The model under review builds one solid part; all positions refer to its coordinate system, in mm. Face numbers are marked on the shaded views. A direction names the side the tool comes from. Give positions to 0.01 mm unless a question says otherwise; leave off trailing zeros. Loops run counter-clockwise (first coordinate to the right, second up) from the corner with the lowest first, then second, coordinate; pieces in that order, holes last. Notation, with made-up numbers: (3.5, 16.25) - (49.5, 16.25) arc R26 cw to (49.5, 47.25) - close; hole circle Ø2 at (17, 69). An arc over 180 degrees is marked (long way). Answer as a JSON object with one key per item and string values.
from build123d import *

# Parameters (mm, degrees)
BOSS_EXTRUDE2_DEPTH      = 10
SKETCH3_R                = 3
BOSS_EXTRUDE3_DEPTH      = 100
BOSS_EXTRUDE3_DEPTH_BACK = 110
BOSS_EXTRUDE4_DEPTH      = 3
BOSS_EXTRUDE5_DEPTH      = 3
BOSS_EXTRUDE6_DEPTH      = 3
CUT_EXTRUDE1_REACH       = 22
SKETCH9_W                = 10
SKETCH9_H                = 0.75


with BuildPart() as part:
    # Sketch1 → Boss-Extrude2 (new body)
    with BuildSketch(Plane.XY):
        with BuildLine():
            Line((5, 100), (5, 0))
            Line((5, 0), (5, -10))
            Line((5, -10), (-5, -10))
            Line((-5, -10), (-5, 0))
            Line((-5, 0), (-5, 100))
            ThreePointArc((-5, 100), (0, 105), (5, 100))
        make_face()
        with BuildLine():
            Line((-2.5, 0), (-2.5, 100))
            ThreePointArc((-2.5, 100), (0, 102.5), (2.5, 100))
            Line((2.5, 100), (2.5, 0))
            ThreePointArc((2.5, 0), (0, -2.5), (-2.5, 0))
        make_face(mode=Mode.SUBTRACT)
    extrude(amount=BOSS_EXTRUDE2_DEPTH)

    # Sketch3 → Boss-Extrude3 (add, two sides)
    with BuildSketch(Plane(origin=(5, 0, 0), x_dir=(0, 0, -1), z_dir=(1, 0, 0))) as boss_extrude3_sk:
        with Locations((-5, -6.25)):
            Circle(SKETCH3_R)
    extrude(amount=BOSS_EXTRUDE3_DEPTH)
    extrude(boss_extrude3_sk.sketch, amount=-BOSS_EXTRUDE3_DEPTH_BACK)

    # Sketch6 → Boss-Extrude4 (add)
    with BuildSketch(Plane(origin=(0, -9.25, 0), x_dir=(-1, 0, 0), z_dir=(0, -1, 0))):
        Polygon((-105, -2), (-105, 10), (-135, 10), (-135, -20), (-105, -20), (-105, -8), align=None)
        Polygon((105, -2), (105, 10), (135, 10), (135, -20), (105, -20), (105, -8), align=None)
    extrude(amount=-BOSS_EXTRUDE4_DEPTH)

    # Sketch7 → Boss-Extrude5 (add)
    with BuildSketch(Plane(origin=(0, -6.25, 0), x_dir=(1, 0, 0), z_dir=(0, 1, 0))):
        Polygon((-105, -2), (-105, 10), (-135, 10), (-135, -20), (-105, -20), (-105, -8), align=None)
        Polygon((-108, -2), (-108, 7), (-132, 7), (-132, -17), (-108, -17), (-108, -8), align=None, mode=Mode.SUBTRACT)
    extrude(amount=BOSS_EXTRUDE5_DEPTH)

    # Sketch8 → Boss-Extrude6 (add)
    with BuildSketch(Plane(origin=(0, -6.25, 0), x_dir=(1, 0, 0), z_dir=(0, 1, 0))):
        Polygon((135, -2), (135, 10), (105, 10), (105, -20), (135, -20), (135, -8), align=None)
        Polygon((132, -2), (132, 7), (108, 7), (108, -17), (132, -17), (132, -8), align=None, mode=Mode.SUBTRACT)
    extrude(amount=BOSS_EXTRUDE6_DEPTH)

    # Sketch9 → Cut-Extrude1 (cut, up to next)
    with BuildSketch(Plane.XY.offset(10), mode=Mode.PRIVATE) as cut_extrude1_sk1:
        with Locations((0, -9.625)):
            Rectangle(SKETCH9_W, SKETCH9_H)
    cut_extrude1_tool1 = extrude(cut_extrude1_sk1.sketch, amount=-CUT_EXTRUDE1_REACH, mode=Mode.PRIVATE) & part.part
    add(cut_extrude1_tool1.solids().sort_by_distance((0, -9.625, 10))[0], mode=Mode.SUBTRACT)


solid = part.part
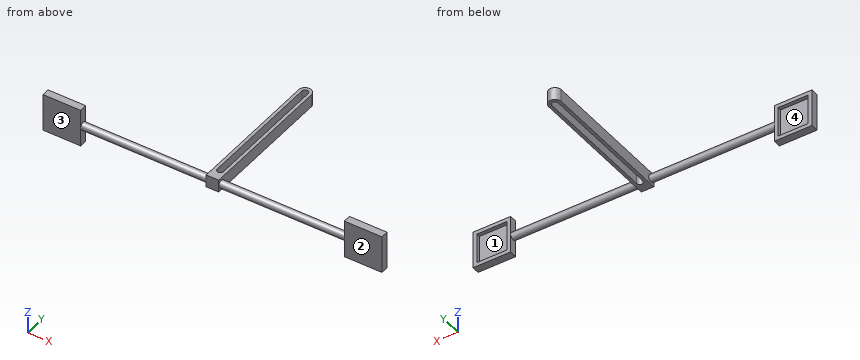
Q1. The part is to be moulded in two halves that separate along X. For the marked faces 3 and 4, say which applies: +X half, -X half, draft (parallel to the pull), parting line (faces both ways), or undercut.
Results:
{"face 3": "draft", "face 4": "undercut"}
Q2. For the marked faces 1 and 2, list the 3-axis set-ups (+Z, -Z, +X, -X, +Y, -Y) from which the entire face can be reached by the end or side of a thin tool; tool diameter is ignored.
Results:
{"face 1": "+Y", "face 2": "+Z, -Z, +X, -X, -Y"}
Q3. To check wall thickness, follow probe 1 along X at (y, z) = (31.5, 1.5); probe 2 along X at (y, z) = (-4, 17.25); probe 3 along Y at (x, z) = (116, 17.5). State the ranges of each line that lie inside material, in increasing order. Write a range as [from, to].
Results:
{"probe 1": "x = [-5, -2.5], [2.5, 5]", "probe 2": "x = [-135, -105], [105, 135]", "probe 3": "y = [-9.25, -3.25]"}
Q4. Clearance check with flat-ended pins moving along their axes: pin 1 Ø12 at (y, z) = (20, -0.5) entering from +X; pin 2 Ø12 at (x, y) = (29, 6) entering from -Z; pin 3 Ø12 at (x, z) = (123, 5.5) entering from +Y; pin 4 Ø8 at (x, z) = (-15.5, 4) entering from -Y. State where each tip first meets the part, or that it passes through.
Results:
{"pin 1": "stops at x = 5", "pin 2": "passes through", "pin 3": "stops at y = -6.25", "pin 4": "stops at y = -9.25"}
Q5. Consider section A-A, the plane x = 0. State the section outline as (y, z) points, plus the area to 3 significant figures.
Results:
{"outline": "(-9.25, 0) - (-2.5, 0) - (-2.5, 10) - (-9.25, 10) - close; (102.5, 0) - (105, 0) - (105, 10) - (102.5, 10) - close", "area": "92.5 mm^2"}
Q6. Consider section B-B, the plane z = 14. State the section outline as (x, y) points.
Results:
{"outline": "(-135, -9.25) - (-105, -9.25) - (-105, -3.25) - (-108, -3.25) - (-108, -6.25) - (-132, -6.25) - (-132, -3.25) - (-135, -3.25) - close; (105, -9.25) - (135, -9.25) - (135, -3.25) - (132, -3.25) - (132, -6.25) - (108, -6.25) - (108, -3.25) - (105, -3.25) - close"}
Q7. Consider section C-C, the plane y = 95.5. State the section outline as (x, z) points.
Results:
{"outline": "(-5, 0) - (-2.5, 0) - (-2.5, 10) - (-5, 10) - close; (2.5, 0) - (5, 0) - (5, 10) - (2.5, 10) - close"}
